Source: three-view drawing plus pictorial views. Frame: mm from the lowest corner of the part. A direction names the side the tool comes from. Give positions to 0.01 mm unless a question says otherwise; leave off trailing zeros. Order: outer loops, then holes, each group sorted by start corner. A loop starts at its lowest first (then second) coordinate and runs counter-clockwise, first axis right, second up. Notation, with made-up numbers: M -18.75,34 L 11.25,34 A11 cw 11.25,52 Z; hole C 25.25,-30.75 d8. An arc over 180 degrees is marked long. Use CSV: the item, a comma, the result in double quotes.
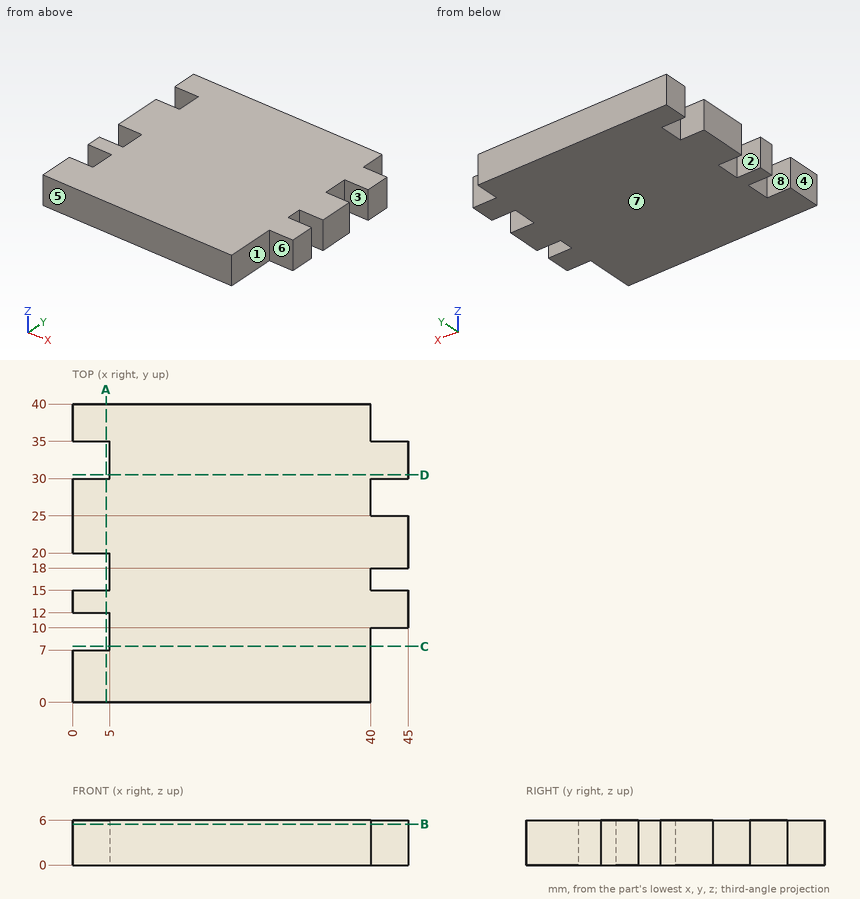
1. Reachability of the marked faces 1, 2, 3, 4 and 5 from +Z, -Z, +X, -X, +Y, -Y: full face, straight path, thin tool, end or side. Return the list, or none.
Answer:
face 1,"+Z, -Z, +X, -Y"
face 2,"+Z, -Z, -X"
face 3,"+Z, -Z, +X"
face 4,"+Z, -Z, -X, +Y, -Y"
face 5,"+Z, -Z, +X, -X, -Y"
2. Section A-A, the plane x = 4.5. Return the cut outline in (y, z).
Answer:
outline,"M 0,0 L 7,0 L 7,6 L 0,6 Z; M 12,0 L 15,0 L 15,6 L 12,6 Z; M 20,0 L 30,0 L 30,6 L 20,6 Z; M 35,0 L 40,0 L 40,6 L 35,6 Z"
3. Section C-C, the plane y = 7.5. Return the cut outline in (x, z), plus the area to 3 significant figures.
Answer:
outline,"M 5,0 L 40,0 L 40,6 L 5,6 Z"
area,"210 mm2"
4. Pin query (flat end, axial travel): pin 1 Ø2.5 at (y, z) = (8.5, 2.5) entering from -X; pin 2 Ø2.5 at (x, z) = (41.5, 4) entering from -Y; pin 3 Ø1.5 at (y, z) = (17, 3.5) entering from +X. Return the tip coordinate at first contact, or that it passes through.
Answer:
pin 1,"x = 5"
pin 2,"y = 10"
pin 3,"x = 40"
5. Pull-direction query (Y, two-part tool) for the marked faces 6, 7 and 8; classes: +Y half, -Y half, draft (parallel to the pull), parting line (faces both ways), or undercut.
Answer:
face 6,"-Y half"
face 7,"draft"
face 8,"undercut"
6. Line query: line 1 (Y direction, x = 41.5, z = 4.9); line 2 (X direction, y = 38, z = 4); line 3 (X direction, y = 7.5, z = 4.65). Output: solid intervals per line, ascending.
Answer:
line 1,"10 to 15, 18 to 25, 30 to 35"
line 2,"0 to 40"
line 3,"5 to 40"
7. Section D-D, the plane y = 30.5. Return the cut outline in (x, z).
Answer:
outline,"M 5,0 L 45,0 L 45,6 L 5,6 Z"
8. Section B-B, the plane z = 5.5. Return the cut outline in (x, y), plus the area to 3 significant figures.
Answer:
outline,"M 0,0 L 40,0 L 40,10 L 45,10 L 45,15 L 40,15 L 40,18 L 45,18 L 45,25 L 40,25 L 40,30 L 45,30 L 45,35 L 40,35 L 40,40 L 0,40 L 0,35 L 5,35 L 5,30 L 0,30 L 0,20 L 5,20 L 5,15 L 0,15 L 0,12 L 5,12 L 5,7 L 0,7 Z"
area,"1,610 mm2"
